Answer from the drawing. Dimensions are ordinates in mm from the lowest x, y and z of the part. A direction names the side the tool comes from. Give positions to 0.01 mm unless a question says otherwise; leave off trailing zeros. Order: outer loops, then holes, each group sorted by start corner. A loop starts at its lowest first (then second) coordinate and runs counter-clockwise, first axis right, second up. Notation, with made-up numbers: (29.5, 11.5) - (44.5, 11.5) arc R14 cw to (44.5, 15.5) - close; hole circle Ø1 at (59, 41). An arc over 180 degrees is marked (long way). Answer in a Markdown table with one row per item. Add a question column.
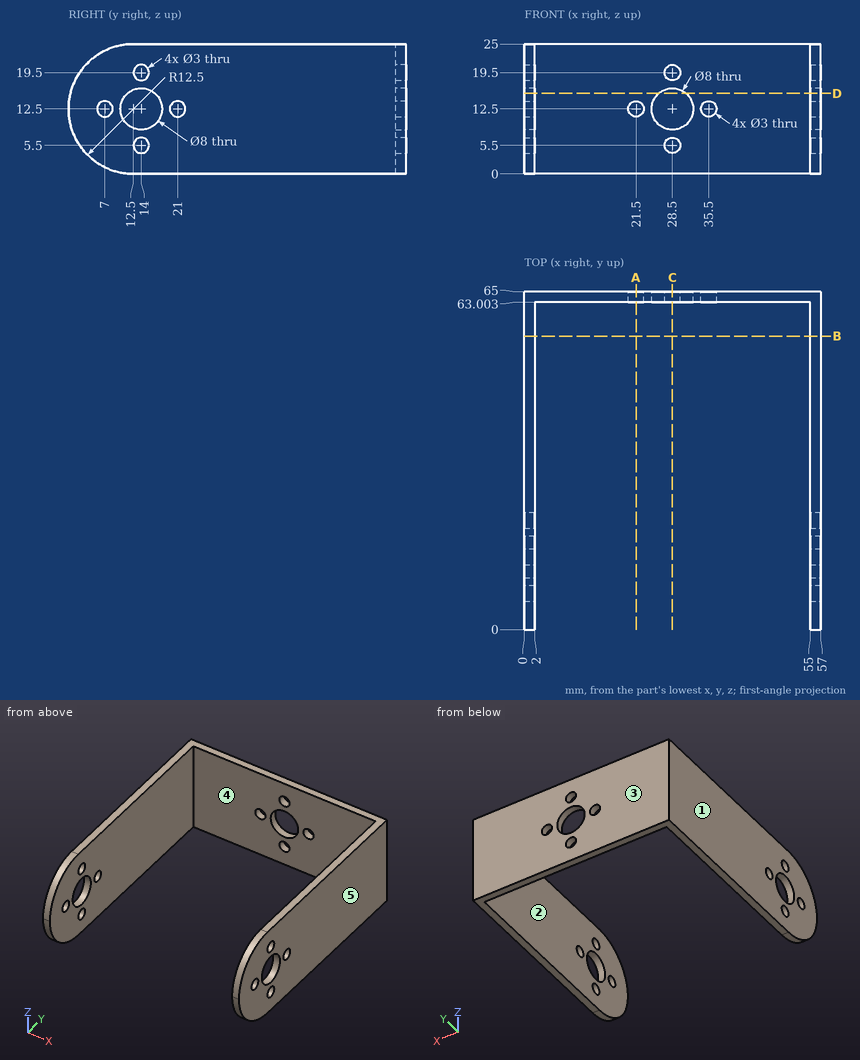
(1) Straight lines are drawn through the part: line 1 (X direction, y = 64.45, z = 12.5); line 2 (Z direction, x = 1, y = 14); line 3 (X direction, y = 45.5, z = 22.5). For each, find the intervals that lie inside material, in ascending order.
(2) Find section D-D, the plane z = 15.5. Write down the section's boundary in (x, y) (1 decimal).
(3) Find section A-A, the plane x = 21.5. Write down the section's boundary in (y, z).
(4) For the marked faces 1 and 2, determine the directions among +Z, -Z, +X, -X, +Y, -Y from which every point of the face is accessible in a straight line to the end or side of a thin tool.
(5) The mould has two halves that part along X. Classify the marked faces 3, 4 and 5: +X half, -X half, draft (parallel to the pull), parting line (faces both ways), or undercut.
(6) Find section C-C, the plane x = 28.5. Write down the section's boundary in (y, z).
(7) Each of these flat-tipped pins is pushed along its axis until it touches: P1, Ø3.5, axis at x = 21.5, z = 12.5, coming from the -Y side; P2, Ø12, axis at x = 7.5, y = 9, coming from the +Z side. Where does it stop, or does it pass through?
(8) Find section B-B, the plane y = 56.5. Write down the section's boundary in (x, z), plus the area to 3 significant figures.
Answer key:
| question | item | result |
|---|---|---|
| 1 | line 1 | 0 to 20, 23 to 24.5, 32.5 to 34, 37 to 57 |
| 1 | line 2 | 0 to 4, 7 to 8.5, 16.5 to 18, 21 to 25 |
| 1 | line 3 | 0 to 2, 55 to 57 |
| 2 | outline | (0, 0.4) - (2, 0.4) - (2, 11.4) - (0, 11.4) - close; (0, 16.6) - (2, 16.6) - (2, 63) - (25.9, 63) - (25.9, 65) - (0, 65) - close; (31.1, 63) - (55, 63) - (55, 16.6) - (57, 16.6) - (57, 65) - (31.1, 65) - close; (55, 0.4) - (57, 0.4) - (57, 11.4) - (55, 11.4) - close |
| 3 | outline | (63, 0) - (65, 0) - (65, 11) - (63, 11) - close; (63, 14) - (65, 14) - (65, 25) - (63, 25) - close |
| 4 | face 1 | +Z, -Z, -X, +Y, -Y |
| 4 | face 2 | +Z, -Z, -Y |
| 5 | face 3 | draft |
| 5 | face 4 | undercut |
| 5 | face 5 | +X half |
| 6 | outline | (63, 0) - (65, 0) - (65, 4) - (63, 4) - close; (63, 7) - (65, 7) - (65, 8.5) - (63, 8.5) - close; (63, 16.5) - (65, 16.5) - (65, 18) - (63, 18) - close; (63, 21) - (65, 21) - (65, 25) - (63, 25) - close |
| 7 | P1 | y = 63 |
| 7 | P2 | z = 24.95 |
| 8 | outline | (0, 0) - (2, 0) - (2, 25) - (0, 25) - close; (55, 0) - (57, 0) - (57, 25) - (55, 25) - close |
| 8 | area | 100 mm² |
